Read the model definition and answer for the solid it produces. Units are mm, in the model's axes. Face numbers are marked on the shaded views. A direction names the side the tool comes from. Give positions to 0.01 mm unless a question says otherwise; leave off trailing zeros. Order: outer loops, then holes, each group sorted by start corner. A loop starts at its lowest first (then second) coordinate and runs counter-clockwise, first axis right, second up.
Autodesk Inventor part; units mm, degrees
ref_plane "YZ Plane" through (0, 0, 0) normal (1, 0, 0) x (0, 1, 0)
ref_plane "XZ Plane" through (0, 0, 0) normal (0, 1, 0) x (-1, 0, 0)
ref_plane "XY Plane" through (0, 0, 0) normal (0, 0, 1) x (1, 0, 0)
sketch "Sketch1" plane through (0, 0, 0) normal (0, 1, 0) x (-1, 0, 0)
  line L0 (14.2, 15.6875) -> (-5.8, 15.6875)
  line L1 (-5.8, 15.6875) -> (-5.8, -7.3125)
  line L2 (-5.8, -7.3125) -> (14.2, -7.3125)
  line L3 (14.2, -7.3125) -> (14.2, 15.6875)
  circle A0 centre (4.2, 4.1875) radius 2.75
  point P0 (0, 0)
  dimension "d0" = 20
  dimension "d1" = 23
  dimension "d9" = 5.5
  dimension "d10" = 11.5
  dimension "d11" = 10
extrude "Extrusion2" add sketch "Sketch1" along normal blind 3
sketch "Sketch3" plane through (0, 3, 0) normal (0, 1, 0) x (1, 0, 0)
  line L0 (5.8, -15.6875) -> (5.8, 7.3125)
  line L1 (-14.2, -15.6875) -> (5.8, -15.6875)
  line L2 (5.8, -12.6875) -> (-14.2, -12.6875)
  line L3 (-14.2, -12.6875) -> (-14.2, -15.6875)
  line L4 (-14.2, -15.6875) -> (5.8, -15.6875)
  line L5 (5.8, -15.6875) -> (5.8, -12.6875)
  line L6 (5.8, 7.3125) -> (-14.2, 7.3125)
  line L7 (5.8, 4.3125) -> (-14.2, 4.3125)
  line L8 (-14.2, 4.3125) -> (-14.2, 7.3125)
  line L9 (-14.2, 7.3125) -> (5.8, 7.3125)
  line L10 (5.8, 7.3125) -> (5.8, 4.3125)
  point P0 (0, 0)
  dimension "d14" = 3
  dimension "d15" = 3
extrude "Extrusion3" add sketch "Sketch3" along normal blind 20
sketch "Sketch4" plane through (-14.2, 0, 15.6875) normal (0, 0, 1) x (1, 0, 0)
  circle A0 centre (10, 8) radius 2.75
  circle A1 centre (10, 18) radius 2.75
  line L0 (0, 0) -> (20, 0)
  line L1 (0, 23) -> (20, 23)
  line L2 (20, 0) -> (20, 23)
  line L3 (0, 3) -> (20, 3)
  point P0 (14.2, 0)
  dimension "d18" = 5.5
  dimension "d19" = 5.5
  dimension "d21" = 5
  dimension "d22" = 10
  dimension "d25" = 5
extrude "Extrusion4" cut sketch "Sketch4" against normal through all
fillet "Fillet1" radius 1 24 edges at (-14.2, 3, 4.1875) (-14.2, 13, -4.3125) (5.8, 3, 4.1875) (-14.2, 0, 4.1875) (-14.2, 11.5, -7.3125) (-14.2, 23, -5.8125) (5.8, 23, -5.8125) (-14.2, 23, 14.1875) (-4.2, 23, 12.6875) (-14.2, 13, 12.6875) (-4.2, 23, -4.3125) (-4.2, 23, -7.3125) (5.8, 13, -4.3125) (5.8, 11.5, -7.3125) (5.8, 0, 4.1875) (5.8, 11.5, 15.6875) (5.8, 13, 12.6875) (-4.2, 23, 15.6875) (5.8, 23, 14.1875) (-14.2, 11.5, 15.6875) (-4.2, 0, 15.6875) (-4.2, 0, -7.3125) (-4.2, 3, 12.6875) (-4.2, 3, -4.3125)
properties part number "top printhead screwplate2"
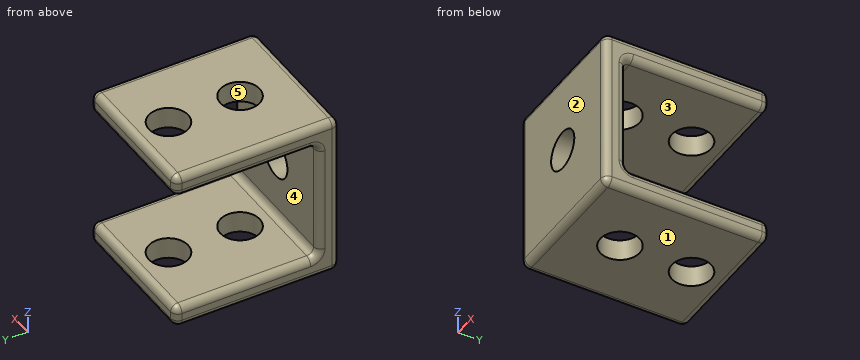
1) The part is cut by section B-B on y = 11.75. Determine the outline of the cut face in (x, z).
Final values:
outline: (-14.2, -6.31) arc R1 ccw to (-13.2, -7.31) - (4.8, -7.31) arc R1 ccw to (5.8, -6.31) - (5.8, -5.31) arc R1 ccw to (4.8, -4.31) - (-13.2, -4.31) arc R1 ccw to (-14.2, -5.31) - close; (-14.2, 13.69) arc R1 ccw to (-13.2, 12.69) - (4.8, 12.69) arc R1 ccw to (5.8, 13.69) - (5.8, 14.69) arc R1 ccw to (4.8, 15.69) - (-13.2, 15.69) arc R1 ccw to (-14.2, 14.69) - close
2) The part is cut by section C-C on z = 8.75. Determine the outline of the cut face in (x, y), and give its area (3 significant figures).
Final values:
outline: (-14.2, 1) arc R1 ccw to (-13.2, 0) - (4.8, 0) arc R1 ccw to (5.8, 1) - (5.8, 2) arc R1 ccw to (4.8, 3) - (-13.2, 3) arc R1 ccw to (-14.2, 2) - close
area: 59.1 mm2
3) The part is cut by section D-D on x = -4.2. Count the separate pieces of the cut face and the enclosed holes in it, and give its area (3 significant figures).
Final values:
separate pieces: 6
enclosed holes: 0
area: 106 mm2
4) Given pin 1 (3.5 mm diameter, centred on x = -4.2, z = 4.19, fed in from +Y); pin 2 (5 mm diameter, centred on x = -8, z = 2.5, fed in from +Y); pin 3 (12 mm diameter, centred on x = -1, z = 6.5, fed in from +Y), each flat-ended and moving along its own axis, determine where each tip first touches the part or whether it passes through.
Final values:
pin 1: passes through
pin 2: stops at y = 3
pin 3: stops at y = 3.42
5) Consider L1, parallel to Y at x = -4.2, z = -5.65; L2, parallel to Z at x = -3.25, y = 21.5; L3, parallel to Y at x = 3.75, z = 7. Determine where each line is inside the solid, lowest interval first.
Final values:
L1: y = 0 to 5.25, 10.75 to 15.25, 20.75 to 23
L2: z = -7.31 to -4.31, 12.69 to 15.69
L3: y = 0 to 3
6) For a pull along Z with two mould halves and no side action, classify the marked faces 1, 2 and 3 as released by +Z, released by -Z, zero draft, split by the parting line, or undercut.
Final values:
face 1: released by -Z
face 2: zero draft
face 3: undercut
7) A tool of negligible diameter and unlimited length cuts with its end or side. For the marked faces 4 and 5, from which of +Z, -Z, +X, -X, +Y, -Y can it reach the whole face along a straight path? Write none if from no direction.
Final values:
face 4: +X, -X, +Y
face 5: +Z, -Z
8) The part is cut by section A-A on y = 8. Determine the outline of the cut face in (x, z), and give its area (3 significant figures).
Final values:
outline: (-14.2, -6.31) arc R1 ccw to (-13.2, -7.31) - (-6.95, -7.31) - (-6.95, -4.31) - (-13.2, -4.31) arc R1 ccw to (-14.2, -5.31) - close; (-14.2, 13.69) arc R1 ccw to (-13.2, 12.69) - (-6.95, 12.69) - (-6.95, 15.69) - (-13.2, 15.69) arc R1 ccw to (-14.2, 14.69) - close; (-1.45, -7.31) - (4.8, -7.31) arc R1 ccw to (5.8, -6.31) - (5.8, -5.31) arc R1 ccw to (4.8, -4.31) - (-1.45, -4.31) - close; (-1.45, 12.69) - (4.8, 12.69) arc R1 ccw to (5.8, 13.69) - (5.8, 14.69) arc R1 ccw to (4.8, 15.69) - (-1.45, 15.69) - close
area: 85.3 mm2
